Part print with two shaded views. Sizes in mm from the minimum x, y, z corner. A direction names the side the tool comes from. Round coordinates to 2 decimals unless told otherwise and drop trailing zeros. Write each loop counter-clockwise with the first axis right and the second up, starting at its lowest first coordinate (ties: lowest second). Pieces come first, ordered by that corner, then holes. Notation, with made-up numbers: (-23, 23) - (10, 23) arc R25 ccw to (10, 36) - close; hole circle Ø2 at (64.25, 22). An arc over 180 degrees is marked (long way). Use one line per item in the form item = value. Start each with the question number.
Item 1: Drill centre lines: L1, parallel to X at y = 3.85, z = 5.75; L2, parallel to Y at x = 8.25, z = 6 (1 decimal); L3, parallel to X at y = 5.25, z = 5 (1 decimal). Where is each one in solid material? Low to high.
Item 2: Band-saw the part on C-C, the plane y = 2.85. List the corners of the cut face in (x, z).
Item 3: Pin check, flat tips, straight feed: pin 1 (2 mm diameter, centred on y = 3, z = 5.5, fed in from -X); pin 2 (0.7 mm diameter, centred on x = 12, y = 3, fed in from +Z) (3 decimals); pin 3 (3 mm diameter, centred on x = 7, z = 4, fed in from -Y); pin 4 (4 mm diameter, centred on x = 5, z = 5, fed in from +Y). Stop position of each tip, or through.
Item 4: Tool access for the marked faces 1 and 2: list every direction of +Z, -Z, +X, -X, +Y, -Y with a clear straight run to the whole face (end or side of a thin tool).
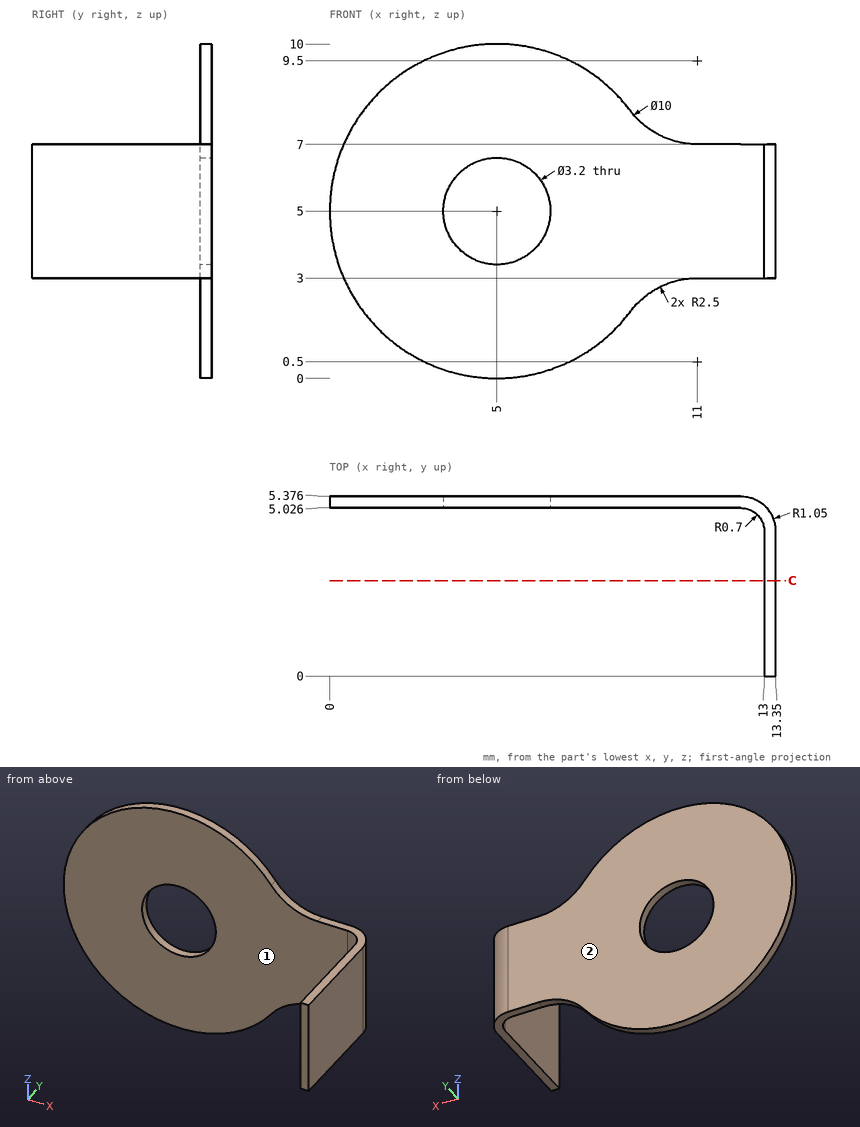
Determined:
q1.L1 = 13 to 13.35
q1.L2 = 5 to 5.4
q1.L3 = 0 to 3.4, 6.6 to 12.8
q2.outline = (13, 3) - (13.35, 3) - (13.35, 7) - (13, 7) - close
q3.pin_1 = 13
q3.pin_2 = through
q3.pin_3 = 5.03
q3.pin_4 = 5.38
q4.face_1 = +Z, -Z, -X, -Y
q4.face_2 = +Z, -Z, +X, -X, +Y
